Work out the finished part from the listing and answer in its coordinate system (mm). A direction names the side the tool comes from. Round coordinates to 2 decimals unless told otherwise and drop trailing zeros. Write each loop counter-clockwise with the first axis right and the second up, starting at its lowest first coordinate (ties: lowest second). Pieces come first, ordered by that corner, then holes.
1. Find section A-A (y = -3.5). Write down the section's boundary in (x, z).
2. Find section B-B (z = 54). Write down the section's boundary in (x, y).
3. Straight lines are drawn through the part: probe 1 along X at (y, z) = (-19.7, 234); probe 2 along X at (y, z) = (-15.5, 36); probe 3 along Y at (x, z) = (5, 121.5). For each, find the intervals that lie inside material, in ascending order.
4. Determine the mould class of faces 4 (the face through (10, -19, 126)), 5 (the face through (19.49, -9.66, 56.63)), 6 (the face through (9.2, -19.6, 0)) for opening direction Z: pulls with the +Z half, pulls with the -Z half, needs draft (parallel to the pull), parting line crosses it, or undercut.
5. A tool of negligible diameter and unlimited length cuts with its end or side. For faces 1 (the face through (1, -10, 126)), 2 (the face through (19.493, -7.897, 7.388)), 3 (the face through (10.264, -19.507, 74.994)), from which of +Z, -Z, +X, -X, +Y, -Y can it reach the whole face along a straight path? Write none if from no direction.
6. A flat-ended cylindrical pin translates along its axis: pin 1 Ø9.5 at (x, z) = (10, 69) entering from -Y. Find the tip coordinate at first contact, or state that the pin passes through.
```python
from build123d import *

# Parameters (mm, degrees)
SKETCH_1_W          = 20
SKETCH_1_H          = 20
SKETCH_1_W_2        = 18
SKETCH_1_H_2        = 18
EXTRUDE_2_DEPTH     = 255
SKETCH_2_R          = 2.65
SKETCH_2_R_2        = 1.1
CUT_EXTRUDE_1_DEPTH = 20
SKETCH_5_R          = 2.65
CUT_EXTRUDE_2_DEPTH = 20
SKETCH_6_R          = 6
CUT_EXTRUDE_3_DEPTH = 10


with BuildPart() as part:
    # 草图1 → 凸台-拉伸2 (new body)
    with BuildSketch(Plane.XY):
        with Locations((10, -10)):
            Rectangle(SKETCH_1_W, SKETCH_1_H)
        with Locations((10, -10)):
            Rectangle(SKETCH_1_W_2, SKETCH_1_H_2, mode=Mode.SUBTRACT)
    extrude(amount=EXTRUDE_2_DEPTH)

    # 草图2 → 切除-拉伸1 (cut)
    with BuildSketch(Plane(origin=(0, -20, 0), x_dir=(-1, 0, 0), z_dir=(0, -1, 0))):
        with Locations(Location((-10, -9, 0), (0, 0, 90))):
            Circle(SKETCH_2_R)
        with Locations(Location((-10, -24, 0), (0, 0, 90))):
            Circle(SKETCH_2_R)
        with Locations(Location((-10, -39, 0), (0, 0, 90))):
            Circle(SKETCH_2_R)
        with Locations(Location((-10, -54, 0), (0, 0, 90))):
            Circle(SKETCH_2_R)
        with Locations(Location((-10, -69, 0), (0, 0, 90))):
            Circle(SKETCH_2_R)
        with Locations(Location((-10, -99, 0), (0, 0, 90))):
            Circle(SKETCH_2_R_2)
        with Locations(Location((-10, -129, 0), (0, 0, 90))):
            Circle(SKETCH_2_R_2)
        with Locations(Location((-10, -144, 0), (0, 0, 90))):
            Circle(SKETCH_2_R_2)
        with Locations(Location((-10, -174, 0), (0, 0, 90))):
            Circle(SKETCH_2_R_2)
        with Locations(Location((-10, -189, 0), (0, 0, 90))):
            Circle(SKETCH_2_R_2)
        with Locations(Location((-10, -219, 0), (0, 0, 90))):
            Circle(SKETCH_2_R_2)
        with Locations(Location((-10, -234, 0), (0, 0, 90))):
            Circle(SKETCH_2_R_2)
        with Locations(Location((-10, -249, 0), (0, 0, 90))):
            Circle(SKETCH_2_R_2)
        with Locations(Location((-10, -84, 0), (0, 0, 90))):
            Circle(SKETCH_2_R_2)
    extrude(amount=-CUT_EXTRUDE_1_DEPTH, mode=Mode.SUBTRACT)

    # 草图5 → 切除-拉伸2 (cut)
    with BuildSketch(Plane.ZY):
        with Locations(Location((9, -10, 0), (0, 0, 270))):
            Circle(SKETCH_5_R)
        with Locations(Location((24, -10, 0), (0, 0, 270))):
            Circle(SKETCH_5_R)
        with Locations(Location((39, -10, 0), (0, 0, 270))):
            Circle(SKETCH_5_R)
        with Locations(Location((54, -10, 0), (0, 0, 270))):
            Circle(SKETCH_5_R)
    extrude(amount=-CUT_EXTRUDE_2_DEPTH, mode=Mode.SUBTRACT)

    # 草图6 → 切除-拉伸3 (cut)
    with BuildSketch(Plane(origin=(0, -20, 0), x_dir=(-1, 0, 0), z_dir=(0, -1, 0))):
        with Locations(Location((-10, -39, 0), (0, 0, 90))):
            Circle(SKETCH_6_R)
        with Locations(Location((-10, -54, 0), (0, 0, 90))):
            Circle(SKETCH_6_R)
        with Locations(Location((-10, -69, 0), (0, 0, 90))):
            Circle(SKETCH_6_R)
    extrude(amount=-CUT_EXTRUDE_3_DEPTH, mode=Mode.SUBTRACT)


solid = part.part
```
Worked answers:
1. outline: (0, 0) - (1, 0) - (1, 255) - (0, 255) - close; (19, 0) - (20, 0) - (20, 255) - (19, 255) - close
2. outline: (0, -20) - (4, -20) - (4, -19) - (1, -19) - (1, -12.65) - (0, -12.65) - close; (0, -7.35) - (1, -7.35) - (1, -1) - (7.35, -1) - (7.35, 0) - (0, 0) - close; (12.65, -1) - (19, -1) - (19, -7.35) - (20, -7.35) - (20, 0) - (12.65, 0) - close; (16, -20) - (20, -20) - (20, -12.65) - (19, -12.65) - (19, -19) - (16, -19) - close
3. probe 1: x = 0 to 8.9, 11.1 to 20
3. probe 2: x = 0 to 1, 19 to 20
3. probe 3: y = -20 to -19, -1 to 0
4. face 4: needs draft
4. face 5: undercut
4. face 6: pulls with the -Z half
5. face 1: +Z, -Z
5. face 2: +X, -X
5. face 3: -Y
6. pin 1: stops at y = -1
